Part print with two shaded views. Sizes in mm from the minimum x, y, z corner. Round coordinates to 2 decimals unless told otherwise and drop trailing zeros. Order: outer loops, then holes, each group sorted by start corner. A loop starts at its lowest first (then second) coordinate and runs counter-clockwise, first axis right, second up. Notation, with made-up numbers: (45.5, 51) - (75.5, 51) arc R27 cw to (75.5, 87) - close; hole circle Ø11 at (40.5, -19.75). An arc over 180 degrees is marked (long way). Write item = value, one per line.
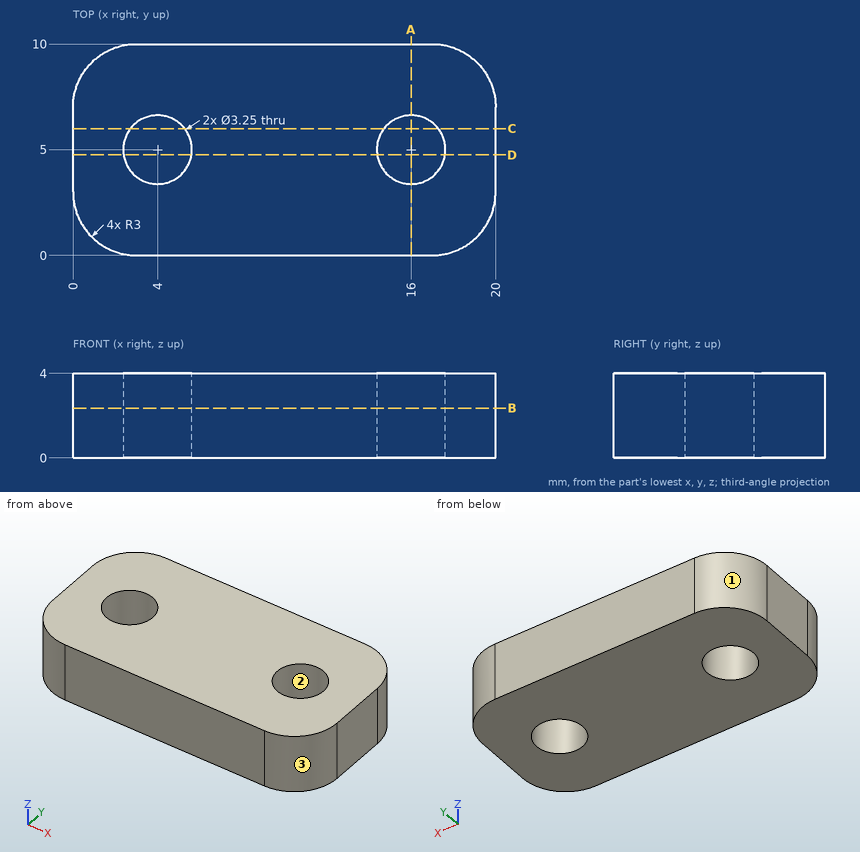
1) Wall check: line 1 along X through (y, z) = (5, 1.5) (1 decimal); line 2 along Y through (x, z) = (4, 1.25) (1 decimal); line 3 along X through (y, z) = (3.75, 3.5). Give the ranges that are in metal, low to high.
Conclusion:
line_1 = 0 to 2.4, 5.6 to 14.4, 17.6 to 20
line_2 = 0 to 3.4, 6.6 to 10
line_3 = 0 to 2.96, 5.04 to 14.96, 17.04 to 20
2) Cut at A-A (x = 16). Write the cut outline in (y, z) (1 decimal).
Conclusion:
outline = (0, 0) - (3.4, 0) - (3.4, 4) - (0, 4) - close; (6.6, 0) - (10, 0) - (10, 4) - (6.6, 4) - close
3) Cut at B-B (z = 2.35). Give the number of separate pieces and of enclosed holes in the cut face, and give its area (3 significant figures).
Conclusion:
separate_pieces = 1
enclosed_holes = 2
area = 176 mm^2
4) Cut at D-D (y = 4.75). Write the cut outline in (x, z) (1 decimal).
Conclusion:
outline = (0, 0) - (2.4, 0) - (2.4, 4) - (0, 4) - close; (5.6, 0) - (14.4, 0) - (14.4, 4) - (5.6, 4) - close; (17.6, 0) - (20, 0) - (20, 4) - (17.6, 4) - close
5) Mould opens along Y. For the marked faces 1, 2 and 3 say: +Y half, -Y half, draft (parallel to the pull), parting line (faces both ways), or undercut.
Conclusion:
face_1 = +Y half
face_2 = undercut
face_3 = -Y half
6) Flat gauge pin, fed straight in: pin 1 Ø3 at (x, y) = (16, 6) entering from -Z. Where does the tip first touch, or does it go through?
Conclusion:
pin_1 = 0
7) Cut at C-C (y = 6). Write the cut outline in (x, z).
Conclusion:
outline = (0, 0) - (2.72, 0) - (2.72, 4) - (0, 4) - close; (5.28, 0) - (14.72, 0) - (14.72, 4) - (5.28, 4) - close; (17.28, 0) - (20, 0) - (20, 4) - (17.28, 4) - close
